Here's how the part is built. I have some questions about the finished solid (model axes, mm). A direction names the side the tool comes from. Coordinates: 2 decimals unless noted, no trailing zeros. Write each loop counter-clockwise with the first axis right and the second up, starting at its lowest first coordinate (ties: lowest second). Pieces come first, ordered by that corner, then holes. Notation, with made-up numbers: (35, 23) -> (92, 23) arc R29 cw to (92, 53) -> close; hole circle Ø1 at (22, 81). An arc over 180 degrees is marked (long way). Put each result on its own line as item: value. Start each with the question number.
Item 1: I want a section at A-A, the plane x = -32.5. List the corners of the cut face in (y, z) for me.
Item 2: I need wall thicknesses on line 1 (Z direction, x = -32.5, y = 58); line 2 (X direction, y = 4, z = -36.5); line 3 (X direction, y = 59.25, z = -142). Which ranges of each line are inside material? Lowest first, please. Write a range as [from, to].
Item 3: I want a section at D-D, the plane z = -53. List the corners of the cut face in (x, y) for me.
Item 4: If we mould it in two halves opening along X, with no side actions, what happens to faces 3 (the face through (-1.804, 29.913, 33.289)), 4 (the face through (-35.752, 56.866, -79.357)), 5 (the face through (-32.129, 63.289, 33.196)), 6 (the face through (-43.556, 56.866, -56.138))? For each: released by +X, released by -X, zero draft, split by the parting line, or undercut.
Item 5: On a 3-axis mill with a long thin cutter (end or side, diameter ignored), from which of +Z, -Z, +X, -X, +Y, -Y can I reach the whole of each face in a straight line? I mean faces 1 (the face through (-10, 0, -45)), 2 (the face through (-52.196, 23.829, -162.289)). Say none if no direction works.
Item 6: For pin 1 (4 mm diameter, centred on x = -39, z = -67, fed in from -Y), with a flat end and sliding along its axis, tell me the tip position at first contact or that it passes through.
Item 7: I want a section at C-C, the plane y = 18.5. List the corners of the cut face in (x, z) for me, then the cut area to 3 significant figures.
Item 8: I want a section at B-B, the plane z = -142. List the corners of the cut face in (x, y) for me, then the cut area to 3 significant figures.
Autodesk Inventor part; units mm, degrees
ref_plane "YZ Plane" through (0, 0, 0) normal (1, 0, 0) x (0, 1, 0)
ref_plane "XZ Plane" through (0, 0, 0) normal (0, 1, 0) x (-1, 0, 0)
ref_plane "XY Plane" through (0, 0, 0) normal (0, 0, 1) x (1, 0, 0)
sketch "Base" plane through (0, 0, 0) normal (0, 1, 0) x (-1, 0, 0)
  line L0 (0, 35) -> (0, -175)
  line L1 (0, -175) -> (65, -175)
  line L2 (65, -175) -> (65, 35)
  line L3 (65, 35) -> (0, 35)
  dimension "d6" = 210
  dimension "d7" = 65
extrude "Extrusion2" add sketch "Base" along normal blind 65
sketch "Top" plane through (0, 65, 0) normal (0, 1, 0) x (1, 0, 0)
  circle A0 centre (-32.5, 46) radius 17
  circle A1 centre (-32.5, -2) radius 17
  circle A2 centre (-32.5, 94) radius 17
  circle A3 centre (-32.5, 142) radius 17
  line L0 (0, 175) -> (-65, 175)
  line L1 (-65, 175) -> (-65, -35)
  line L2 (-65, -35) -> (0, -35) construction
  line L3 (-32.5, -35) -> (-32.5, 175) construction
  circle A4 centre (-32.5, -2) radius 15
  circle A5 centre (-32.5, 46) radius 15
  circle A6 centre (-32.5, 94) radius 15
  circle A7 centre (-32.5, 142) radius 15
  point P0 (-32.5, 70)
  dimension "d10" = 34
  dimension "d11" = 34
  dimension "d12" = 34
  dimension "d13" = 34
  dimension "d14" = 48
  dimension "d15" = 48
  dimension "d16" = 48
  dimension "d27" = 30
  dimension "d28" = 30
  dimension "d29" = 30
  dimension "d30" = 30
  dimension "d31" = 24
  dimension "d32" = 105
  dimension "d35" = 33
extrude "Extrusion3" cut sketch "Top" against normal up to next contours A4 | A5 | A6 | A7
sketch "Walls" plane through (0, 0, 0) normal (0, -1, 0) x (1, 0, 0)
  line L0 (-11, 24) -> (-54, 24)
  line L1 (-54, 24) -> (-54, -164)
  line L2 (-54, -164) -> (-11, -164)
  line L3 (-11, -164) -> (-11, 24)
  line L4 (-65, 35) -> (0, 35)
  line L5 (0, -175) -> (-65, -175)
  line L6 (0, 35) -> (0, -175)
  line L7 (-65, -175) -> (-65, 35)
  point P0 (0, 0)
  dimension "d21" = 11
  dimension "d22" = 11
  dimension "d23" = 11
  dimension "d24" = 11
  dimension "d33" = 43
extrude "Extrusion4" cut sketch "Walls" against normal blind 48.5 contours L3 L2 L1 L0
sketch "Sketch6" plane through (0, 0, 35) normal (1, 0, 0) x (0, 0, -1)
  line L0 (0, 0) -> (210, 0)
  line L1 (11, 48.5) -> (199, 48.5)
  point P0 (35, 0)
  point P1 (33.3852, 33.5)
  dimension "d34" = 48.5
fillet "Fillet1" radius 6 8 edges at (-32.5, 65, 35) (-65, 65, -70) (0, 65, -70) (0, 32.5, 35) (-65, 32.5, 35) (0, 32.5, -175) (-32.5, 65, -175) (-65, 32.5, -175)
sketch "Sketch7" plane through (-65, 0, -169) normal (-1, 0, 0) x (0, 0, 1)
  line L0 (0, 59) -> (198, 59)
  line L1 (99, 59) -> (99, 0) construction
  line L2 (0, 0) -> (198, 0)
  circle A0 centre (99, 0) radius 6.35
  point P0 (169, 0)
  dimension "d40" = 12.7
extrude "Extrusion5" cut sketch "Sketch7" against normal up to surface (11 mm away)
fillet "Fillet2" radius 6 4 edges at (-11, 24.25, 24) (-54, 24.25, 24) (-11, 24.25, -164) (-54, 24.25, -164)
sketch "Sketch8" plane through (0, 0, 29) normal (1, 0, 0) x (0, 0, -1)
  line L0 (0, 0) -> (198, 0)
  line L1 (198, 65) -> (0, 65)
  point P0 (29, 0)
  dimension "d42" = 65
fillet "Fillet3" radius 1.5 8 edges at (-52.2426, 48.5, 22.2426) (-32.5, 48.5, 24) (-12.7574, 48.5, 22.2426) (-11, 48.5, -70) (-12.7574, 48.5, -162.2426) (-32.5, 48.5, -164) (-52.2426, 48.5, -162.2426) (-54, 48.5, -70)
equation "\"d8\" = d7"
equation "\"d11\" = d10"
equation "\"d12\" = d10"
equation "\"d13\" = d10"
equation "\"d15\" = d14"
equation "\"d16\" = d14"
equation "\"d28\" = d27"
equation "\"d29\" = d27"
equation "\"d30\" = d27"
equation "\"d22\" = d21"
equation "\"d23\" = d21"
equation "\"d24\" = d23"
equation "\"d25\" = d7 - 1.5 * d21"
equation "\"d41\" = d36"
equation "\"d43\" = 0.25 * d36"
properties part number "Full"
Calculated:
1. outline: (0, -175) -> (59, -175) arc R6 ccw to (65, -169) -> (65, -157) -> (48.5, -157) -> (48.5, -162.5) arc R1.5 cw to (47, -164) -> (0, -164) -> close; (0, 24) -> (47, 24) arc R1.5 cw to (48.5, 22.5) -> (48.5, 17) -> (65, 17) -> (65, 29) arc R6 ccw to (59, 35) -> (0, 35) -> close; (48.5, -127) -> (65, -127) -> (65, -109) -> (48.5, -109) -> close; (48.5, -79) -> (65, -79) -> (65, -61) -> (48.5, -61) -> close; (48.5, -31) -> (65, -31) -> (65, -13) -> (48.5, -13) -> close
2. line 1: z = [-175, -157], [-127, -109], [-79, -61], [-31, -13], [17, 35]
2. line 2: x = [-65, -54], [-11, 0]
2. line 3: x = [-64.99, -47.5], [-17.5, -0.01]
3. outline: (-65, 0) -> (-54, 0) -> (-54, 47) arc R1.5 cw to (-52.5, 48.5) -> (-45.77, 48.5) -> (-45.77, 65) -> (-59, 65) arc R6 ccw to (-65, 59) -> close; (-19.23, 48.5) -> (-12.5, 48.5) arc R1.5 cw to (-11, 47) -> (-11, 0) -> (0, 0) -> (0, 59) arc R6 ccw to (-6, 65) -> (-19.23, 65) -> close
4. face 3: released by +X
4. face 4: undercut
4. face 5: zero draft
4. face 6: undercut
5. face 1: +Z, -Z, +X, -X, -Y
5. face 2: -Y
6. pin 1: stops at y = 48.5
7. outline: (-65, -169) arc R6 ccw to (-59, -175) -> (-6, -175) arc R6 ccw to (0, -169) -> (0, 29) arc R6 ccw to (-6, 35) -> (-59, 35) arc R6 ccw to (-65, 29) -> close; hole (-54, -158) arc R6 ccw to (-48, -164) -> (-17, -164) arc R6 ccw to (-11, -158) -> (-11, 18) arc R6 ccw to (-17, 24) -> (-48, 24) arc R6 ccw to (-54, 18) -> close
7. area: 5,570 mm2
8. outline: (-65, 0) -> (-54, 0) -> (-54, 47) arc R1.5 cw to (-52.5, 48.5) -> (-47.5, 48.5) -> (-47.5, 65) -> (-59, 65) arc R6 ccw to (-65, 59) -> close; (-17.5, 48.5) -> (-12.5, 48.5) arc R1.5 cw to (-11, 47) -> (-11, 0) -> (0, 0) -> (0, 59) arc R6 ccw to (-6, 65) -> (-17.5, 65) -> close
8. area: 1,630 mm2
